Read the model definition and answer for the solid it produces. Units are mm, in the model's axes. A direction names the side the tool comes from. Give positions to 0.01 mm unless a question says otherwise; leave off trailing zeros. Order: outer loops, then holes, each group sorted by start corner. A loop starts at its lowest first (then second) coordinate and runs counter-clockwise, first axis right, second up. Notation, with made-up numbers: (-2, 49.25) -> (44, 49.25) arc R5 ccw to (44, 57.25) -> close; hole circle Ø3 at (-29, -35.5). An arc over 180 degrees is marked (long way). Answer as CSV lines item,"result". Start each with the question number.
1) Find section B-B (x = 5.5). Determine the outline of the cut face in (y, z), and give its area (3 significant figures).
2) Find section C-C (z = 20.5). Determine the outline of the cut face in (x, y), and give its area (3 significant figures).
3) Find section A-A (z = -10.5). Determine the outline of the cut face in (x, y).
4) For faces 4 (the face through (46, -13, -1.708)), 5 (the face through (-33, -45, 26)), 6 (the face through (61.358, -17, 18)), 7 (the face through (11, 0, 15)), 8 (the face through (-18.642, -8, -13)), determine the directions among +Z, -Z, +X, -X, +Y, -Y from which every point of the face is accessible in a straight line to the end or side of a thin tool.
5) Straight lines are drawn through the part: L1, parallel to Z at x = 5, y = -20; L2, parallel to Z at x = 40, y = -16; L3, parallel to Y at x = 39.5, z = 0. For each, find the intervals that lie inside material, in ascending order. Write a range as from..to.
6) Find section D-D (y = -15). Determine the outline of the cut face in (x, z).
7) Flat-ended cylindrical pins translate along their axes: pin 1 Ø3.5 at (x, z) = (-34, 28) entering from -Y; pin 2 Ø2 at (x, y) = (-27.5, -42.5) entering from -Z; pin 3 Ø6.5 at (x, y) = (-2, -8.5) entering from -Z. Find the tip coordinate at first contact, or state that the pin passes through.
8) The mould has two halves that part along X. Classify faces 1 (the face through (-38.642, -17, 15)), 2 (the face through (16.358, -8, -12)), 3 (the face through (18, -60, 33)): +X half, -X half, draft (parallel to the pull), parting line (faces both ways), or undercut.
```python
from build123d import *

# Parameters (mm, degrees)
F3_DEPTH = 60
F5_DEPTH = 60.001
F7_DEPTH = 100.001


with BuildPart() as f3:
    # F2 (on Front) → F3 (new body)
    with BuildSketch(Plane.XZ):
        Polygon((61.358089, 38.292337), (-38.641911, 38.292337), (-38.641911, -21.707663), (-18.641911, -21.707663), (-18.641911, -6.707663), (16.358089, -6.707663), (16.358089, -21.707663), (31.358089, -21.707663), (31.358089, -1.707663), (61.358089, -1.707663), align=None)
    extrude(amount=F3_DEPTH)

    # F4 (on face) → F5 (cut, through all)
    with BuildSketch(Plane(origin=(0, 0, -21.707663), x_dir=(1, 0, 0), z_dir=(0, 0, -1))):
        Polygon((-38.641911, 60), (-38.641911, 45), (-26.710982, 45), (-18.641911, 49.65868), (-18.641911, 60), align=None)
        Polygon((-18.641911, 60), (-18.641911, 49.65868), (-0.730219, 60), align=None)
        Polygon((61.358089, 60), (36.358089, 60), (61.358089, 35), align=None)
    extrude(amount=-F5_DEPTH, mode=Mode.SUBTRACT)

    # F6 (on face) → F7 (cut, through all)
    with BuildSketch(Plane(origin=(-38.641911, 0, 0), x_dir=(0, -1, 0), z_dir=(-1, 0, 0))):
        Polygon((60, -21.707663), (60, 28.292337), (45, 14.655973), (45, -21.707663), align=None)
        Polygon((45, -21.707663), (45, 14.655973), (5, -21.707663), align=None)
    extrude(amount=-F7_DEPTH, mode=Mode.SUBTRACT)


solid = f3.part
```
Findings below:
1,outline,"(-60, 28.29) -> (-21.5, -6.71) -> (0, -6.71) -> (0, 38.29) -> (-60, 38.29) -> close"
1,area,"2,030 mm²"
2,outline,"(-38.64, -45) -> (-26.71, -45) -> (-15.58, -51.43) -> (44.93, -51.43) -> (61.36, -35) -> (61.36, 0) -> (-38.64, 0) -> close"
2,area,"4,900 mm²"
3,outline,"(-38.64, -17.33) -> (-18.64, -17.33) -> (-18.64, 0) -> (-38.64, 0) -> close; (16.36, -17.33) -> (31.36, -17.33) -> (31.36, 0) -> (16.36, 0) -> close"
4,face 4,"-Z, +X, +Y, -Y"
4,face 5,"+Z, -Z, -X, -Y"
4,face 6,"+Z, -Z, +X, +Y, -Y"
4,face 7,"+Z, -Z, +X, -X, +Y"
4,face 8,"-Z, +Y, -Y"
5,L1,"-6.71..38.29"
5,L2,"-1.71..38.29"
5,L3,"-28.88..0"
6,outline,"(-38.64, -12.62) -> (-18.64, -12.62) -> (-18.64, -6.71) -> (16.36, -6.71) -> (16.36, -12.62) -> (31.36, -12.62) -> (31.36, -1.71) -> (61.36, -1.71) -> (61.36, 38.29) -> (-38.64, 38.29) -> close"
7,pin 1,"y = -45"
7,pin 2,"z = 11.47"
7,pin 3,"z = -6.71"
8,face 1,"-X half"
8,face 2,"undercut"
8,face 3,"draft"
